Design review of the part built by this model. Coordinates are the model's own, in mm. Face numbers are marked on the shaded views. A direction names the side the tool comes from. Coordinates: 2 decimals unless noted, no trailing zeros. Write each loop counter-clockwise with the first axis right and the second up, starting at its lowest first coordinate (ties: lowest second). Pieces come first, ordered by that corner, then holes. Notation, with made-up numbers: (50, -32) - (82, -32) arc R18 ccw to (82, -2) - close; hole circle Ø6 at (47.25, -28). An arc over 180 degrees is marked (long way). Use a Markdown table: item, result.
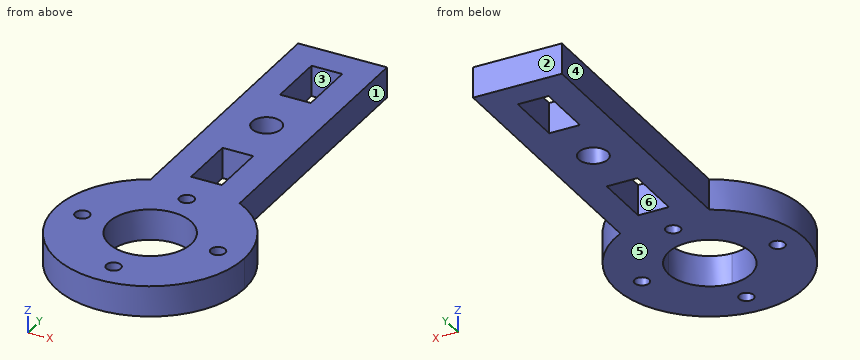
from build123d import *

# Parameters (mm, degrees)
F0_W     = 3.175
F0_H     = 6
F0_R     = 0.75
F1_DEPTH = 3.175


# Not quite as in the source:
# - a length typed as a fraction of an inch, garbled in the dataset ("3 / 203.2 mm" for 3/8 in), is restored


with BuildPart() as f1:
    # F0 (on Top) → F1 (new body)
    with BuildSketch(Plane.XY):
        with BuildLine():
            ThreePointArc((-25.3152321216, 19.8451589555), (-20.7277321216, 20.9918256626), (-16.1402321216, 19.8451589555))
            Line((-16.1402321216, 19.8451589555), (-16.1402321216, 47.9918256626))
            Line((-16.1402321216, 47.9918256626), (-25.3152321216, 47.9918256626))
            Line((-25.3152321216, 47.9918256626), (-25.3152321216, 19.8451589555))
        make_face()
        with Locations((-20.7277321216, 24.9918256626)):
            Rectangle(F0_W, F0_H, mode=Mode.SUBTRACT)
        with BuildLine():
            ThreePointArc((-22.2277321216, 33.4918256626), (-20.7277321216, 34.9918256626), (-19.2277321216, 33.4918256626))
            ThreePointArc((-19.2277321216, 33.4918256626), (-20.7277321216, 31.9918256626), (-22.2277321216, 33.4918256626))
        make_face(mode=Mode.SUBTRACT)
        with Locations((-20.7277321216, 41.9918256626)):
            Rectangle(F0_W, F0_H, mode=Mode.SUBTRACT)
        with BuildLine():
            ThreePointArc((-25.3152321216, 19.8451589555), (-25.744423013, 2.8814840128), (-10.9777321216, 11.2418256626))
            ThreePointArc((-10.9777321216, 11.2418256626), (-12.3673904719, 16.258516554), (-16.1402321216, 19.8451589555))
            ThreePointArc((-16.1402321216, 19.8451589555), (-20.7277321216, 20.9918256626), (-25.3152321216, 19.8451589555))
        make_face()
        with Locations((-27.7277321216, 11.2418256626)):
            Circle(F0_R, mode=Mode.SUBTRACT)
        with Locations((-20.7277321216, 4.2418256626)):
            Circle(F0_R, mode=Mode.SUBTRACT)
        with BuildLine():
            ThreePointArc((-20.7277321216, 6.9918256626), (-23.7329359416, 14.2470294826), (-16.4777321216, 11.2418256626))
            ThreePointArc((-16.4777321216, 11.2418256626), (-17.7225283015, 8.2366218425), (-20.7277321216, 6.9918256626))
        make_face(mode=Mode.SUBTRACT)
        with Locations((-13.7277321216, 11.2418256626)):
            Circle(F0_R, mode=Mode.SUBTRACT)
        with Locations((-20.7277321216, 18.2418256626)):
            Circle(F0_R, mode=Mode.SUBTRACT)
    extrude(amount=F1_DEPTH)


solid = f1.part
(1) Draft analysis for pull direction Y (two halves, no side actions). For the marked faces 1, 2 and 3, state which applies: +Y half, -Y half, draft (parallel to the pull), parting line (faces both ways), or undercut.
Determined:
| item | result |
|---|---|
| face 1 | draft |
| face 2 | +Y half |
| face 3 | undercut |
(2) Take a section at A-A on y = 42. Write out the cut boundary in (x, z) (3 decimals).
Determined:
| item | result |
|---|---|
| outline | (-25.315, 0) - (-22.315, 0) - (-22.315, 3.175) - (-25.315, 3.175) - close; (-19.14, 0) - (-16.14, 0) - (-16.14, 3.175) - (-19.14, 3.175) - close |
(3) For pin 1 (1.8 mm diameter, centred on x = -20.73, y = 33.49, fed in from +Z); pin 2 (1 mm diameter, centred on y = 28.5, z = 1, fed in from -X); pin 3 (1.5 mm diameter, centred on y = 14, z = 1, fed in from -X); pin 4 (1 mm diameter, centred on y = 43, z = 2, fed in from +X), all flat-tipped, find the tip position at first contact; note any pin that passes through.
Determined:
| item | result |
|---|---|
| pin 1 | through |
| pin 2 | x = -25.32 |
| pin 3 | x = -30.27 |
| pin 4 | x = -16.14 |
(4) Take a section at C-C on z = 1.2. State how many separate pieces and enclosed holes the cut face has, and give its area (3 significant figures).
Determined:
| item | result |
|---|---|
| separate pieces | 1 |
| enclosed holes | 8 |
| area | 441 mm2 |
(5) Machinability: for the marked faces 4, 5 and 6, which of the approach directions +Z, -Z, +X, -X, +Y, -Y give a long, thin tool a straight path to every point of the face, cutting with its end or side? Answer none if there is none.
Determined:
| item | result |
|---|---|
| face 4 | +Z, -Z, -X, +Y |
| face 5 | -Z, +X, -X, +Y, -Y |
| face 6 | +Z, -Z |
(6) Take a section at D-D on y = 20.5. Write out the cut boundary in (x, z) (3 decimals).
Determined:
| item | result |
|---|---|
| outline | (-25.315, 0) - (-16.14, 0) - (-16.14, 3.175) - (-25.315, 3.175) - close |
(7) Take a section at B-B on x = -24.5. Write out the cut boundary in (y, z) (1 decimal).
Determined:
| item | result |
|---|---|
| outline | (2.3, 0) - (9.3, 0) - (9.3, 3.2) - (2.3, 3.2) - close; (13.2, 0) - (48, 0) - (48, 3.2) - (13.2, 3.2) - close |
(8) For L1, parallel to X at y = 38.5, z = 3.05; L2, parallel to Y at x = -27.25, z = 1.3; L3, parallel to X at y = 18.5, z = 1.95, list the stretches that pass through material, from the lowest coordinate up. Write a range as from..to.
Determined:
| item | result |
|---|---|
| L1 | -25.32..-16.14 |
| L2 | 3.99..10.66, 11.82..18.49 |
| L3 | -27.24..-21.43, -20.02..-14.22 |
